Source: CAD feature listing. Evaluate the final solid. Frame: model axes, mm. Round coordinates to 2 decimals unless told otherwise and drop trailing zeros. Loops run counter-clockwise (first coordinate to the right, second up) from the corner with the lowest first, then second, coordinate; pieces in that order, holes last. Notation, with made-up numbers: (-23.5, -14.75) -> (-9.5, -14.75) arc R27 ccw to (-9.5, 13.25) -> close; hole circle Ø9 at (11, 4). An arc over 180 degrees is marked (long way). Write item = value, one per line.
from build123d import *

# Parameters (mm, degrees)
L_ANGLE_EQUAL_40X40X3_4_DEPTH = 2000
SKETCH14_R                    = 2
CUT_EXTRUDE1_DEPTH            = 2001.799840064


with BuildPart() as part:
    # Sketch13 → L angle (equal) 40X40X3(4) (new body)
    with BuildSketch(Plane(origin=(0, 0, 0), x_dir=(0, 0, -1), z_dir=(1, 0, 0))):
        with BuildLine():
            Line((0, 40), (0, 0))
            Line((0, 0), (40, 0))
            ThreePointArc((40, 0), (39.121320344, 2.121320344), (37, 3))
            Line((37, 3), (9, 3))
            ThreePointArc((9, 3), (4.757359313, 4.757359313), (3, 9))
            Line((3, 9), (3, 37))
            ThreePointArc((3, 37), (2.121320344, 39.121320344), (0, 40))
        make_face()
    extrude(amount=L_ANGLE_EQUAL_40X40X3_4_DEPTH)

    # Sketch14 → Cut-Extrude1 (cut, through all)
    with BuildSketch(Plane.XY):
        with Locations((1000, 20)):
            Circle(SKETCH14_R)
        with Locations((510, 20)):
            Circle(SKETCH14_R)
        with Locations((1490, 20)):
            Circle(SKETCH14_R)
        with BuildLine():
            Line((2000, 0), (2000, 40))
            Line((2000, 40), (1960, 40))
            Line((1960, 40), (1978.585786438, 21.414213562))
            ThreePointArc((1978.585786438, 21.414213562), (1978.585786438, 18.585786438), (1981.414213562, 18.585786438))
            Line((1981.414213562, 18.585786438), (2000, 0))
        make_face()
        with BuildLine():
            Line((0, 40), (0, 0))
            Line((0, 0), (18.585786438, 18.585786438))
            ThreePointArc((18.585786438, 18.585786438), (21.414213562, 18.585786438), (21.414213562, 21.414213562))
            Line((21.414213562, 21.414213562), (40, 40))
            Line((40, 40), (0, 40))
        make_face()
    extrude(amount=-CUT_EXTRUDE1_DEPTH, mode=Mode.SUBTRACT)


solid = part.part
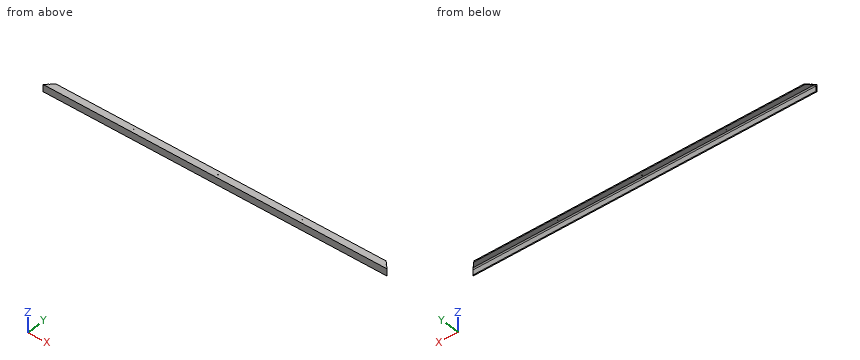
1. Section query A-A (x = 1734). Return the cut outline in (y, z), then the cut area to 3 significant figures.
Evaluation:
outline = (0, -40) arc R3 ccw to (3, -37) -> (3, -9) arc R6 cw to (9, -3) -> (37, -3) arc R3 ccw to (40, 0) -> (0, 0) -> close
area = 235 mm²
2. Contact query for flat-ended pins moving along their axis: pin 1 Ø14 at (x, z) = (1273.5, -26.5) entering from +Y; pin 2 Ø4 at (x, y) = (1534.5, 28.5) entering from -Z. Output: stop coordinate, or through.
Evaluation:
pin_1 = 3
pin_2 = -3
3. Line query: probe 1 along Y at (x, z) = (1603.5, -18.5); probe 2 along Z at (x, y) = (1727.5, 27); probe 3 along X at (y, z) = (3, -8). Output: solid intervals per line, ascending. Write a range as from..to.
Evaluation:
probe_1 = 0..3
probe_2 = -3..0
probe_3 = 3..1997
